```python
from build123d import *

# Parameters (mm, degrees)
SKETCH1_R           = 1.5875
BOSS_EXTRUDE2_DEPTH = 1.6


with BuildPart() as part:
    # Sketch1 → Boss-Extrude2 (new, symmetric)
    with BuildSketch(Plane.XY):
        with BuildLine():
            Line((-149.999999691, 6.4), (149.999999691, 6.4))
            ThreePointArc((149.999999691, 6.4), (156.399999534, -1.57e-07), (149.999999377, -6.4))
            Line((149.999999377, -6.4), (-149.999999377, -6.4))
            ThreePointArc((-149.999999377, -6.4), (-156.4, -1.57e-07), (-149.999999691, 6.4))
        make_face()
        with Locations((-150, 0)):
            Circle(SKETCH1_R, mode=Mode.SUBTRACT)
        with Locations((149.999999534, 0)):
            Circle(SKETCH1_R, mode=Mode.SUBTRACT)
        with BuildLine():
            Line((141.185, 3.2), (-141.185, 3.2))
            ThreePointArc((-141.185, 3.2), (-144.385, 0), (-141.185, -3.2))
            Line((-141.185, -3.2), (141.185, -3.2))
            ThreePointArc((141.185, -3.2), (144.385, 0), (141.185, 3.2))
        make_face(mode=Mode.SUBTRACT)
    extrude(amount=BOSS_EXTRUDE2_DEPTH, both=True)


solid = part.part
```
Design review of the part built by this model. Coordinates are the model's own, in mm. Coordinates: 2 decimals unless noted, no trailing zeros. Loops run counter-clockwise (first coordinate to the right, second up) from the corner with the lowest first, then second, coordinate; pieces in that order, holes last. Notation, with made-up numbers: M -18,-34 L 8,-34 A13 cw 8,-19 Z; hole C 36,-1 d3. An arc over 180 degrees is marked long. One line per question, with ' | ' between items.
(1) We need section B-B (z = 0.05). Give the boundary of the cut face in (x, y) (1 decimal), and give its area (3 significant figures).
Filled in:
outline: M -150,-6.4 L 150,-6.4 A6.4 ccw 150,6.4 L -150,6.4 A6.4 ccw Z; hole C -150,0 d3.2; hole M -141.2,-3.2 L 141.2,-3.2 A3.2 ccw 141.2,3.2 L -141.2,3.2 A3.2 ccw Z; hole C 150,0 d3.2 | area: 2,110 mm^2
(2) We need section A-A (x = 34). Give the boundary of the cut face in (y, z), and give its area (3 significant figures).
Filled in:
outline: M -6.4,-1.6 L -3.2,-1.6 L -3.2,1.6 L -6.4,1.6 Z; M 3.2,-1.6 L 6.4,-1.6 L 6.4,1.6 L 3.2,1.6 Z | area: 20.5 mm^2
(3) Wall thickness on probe 1 along Y at (x, z) = (150, 0.25); probe 2 along Y at (x, z) = (106, -1.4); probe 3 along X at (y, z) = (-1.25, -1.25): over which ranges is each line inside the solid? List them lowest first.
Filled in:
probe 1: y = -6.4 to -1.59, 1.59 to 6.4 | probe 2: y = -6.4 to -3.2, 3.2 to 6.4 | probe 3: x = -156.28 to -150.98, -149.02 to -144.13, 144.13 to 149.02, 150.98 to 156.28
